Source: three-view drawing plus pictorial views. Frame: mm from the lowest corner of the part. Give positions to 0.01 mm unless a question says otherwise; leave off trailing zeros. Order: outer loops, then holes, each group sorted by start corner. A loop starts at its lowest first (then second) coordinate and runs counter-clockwise, first axis right, second up. Notation, with made-up numbers: (17, 7) - (28, 7) arc R32 ccw to (28, 46) - close; hole circle Ø10 at (27.5, 60). An arc over 180 degrees is marked (long way). Use one line per item in the form item = value.
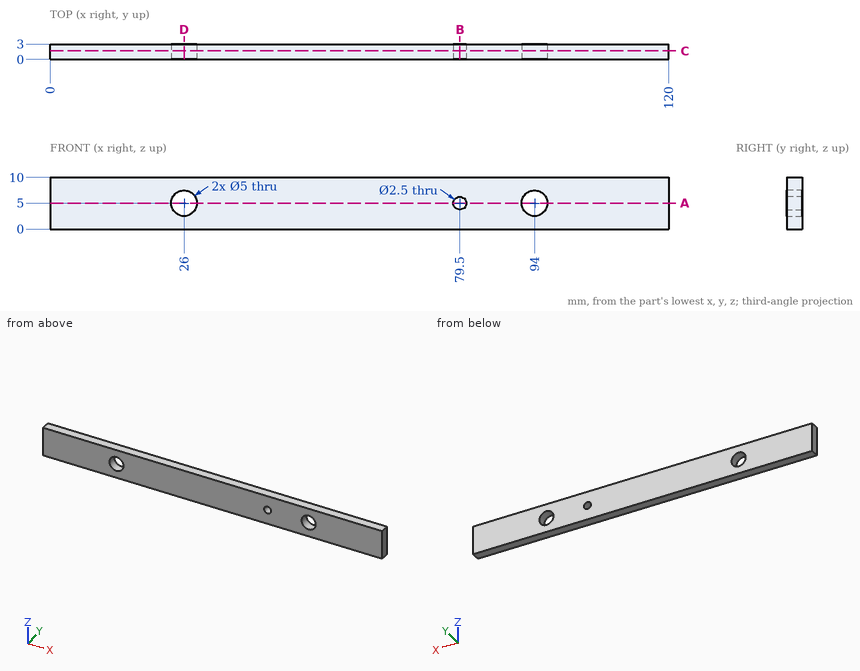
(1) Cut plane A-A on z = 5. Output: boundary loops of the cut face in (x, y).
Computed values:
outline = (0, 0) - (23.5, 0) - (23.5, 3) - (0, 3) - close; (28.5, 0) - (78.25, 0) - (78.25, 3) - (28.5, 3) - close; (80.75, 0) - (91.5, 0) - (91.5, 3) - (80.75, 3) - close; (96.5, 0) - (120, 0) - (120, 3) - (96.5, 3) - close
(2) Ray query, line 1 along X through (y, z) = (1.95, 5); line 2 along Z through (x, y) = (94, 1.85); line 3 along X through (y, z) = (0.35, 6). Return the intervals inside material, ascending.
Computed values:
line_1 = 0 to 23.5, 28.5 to 78.25, 80.75 to 91.5, 96.5 to 120
line_2 = 0 to 2.5, 7.5 to 10
line_3 = 0 to 23.71, 28.29 to 78.75, 80.25 to 91.71, 96.29 to 120
(3) Cut plane B-B on x = 79.5. Output: boundary loops of the cut face in (y, z).
Computed values:
outline = (0, 0) - (3, 0) - (3, 3.75) - (0, 3.75) - close; (0, 6.25) - (3, 6.25) - (3, 10) - (0, 10) - close
(4) Cut plane C-C on y = 1.65. Output: boundary loops of the cut face in (x, z).
Computed values:
outline = (0, 0) - (120, 0) - (120, 10) - (0, 10) - close; hole circle Ø5 at (26, 5); hole circle Ø2.5 at (79.5, 5); hole circle Ø5 at (94, 5)
(5) Cut plane D-D on x = 26. Output: boundary loops of the cut face in (y, z).
Computed values:
outline = (0, 0) - (3, 0) - (3, 2.5) - (0, 2.5) - close; (0, 7.5) - (3, 7.5) - (3, 10) - (0, 10) - close
